Geometry check sheet. Reference: the model listing, model coordinates, mm. A direction names the side the tool comes from. Coordinates: 2 decimals unless noted, no trailing zeros. Write each loop counter-clockwise with the first axis right and the second up, starting at its lowest first coordinate (ties: lowest second). Pieces come first, ordered by that corner, then holes. Notation, with made-up numbers: (76, -8) -> (87, -8) arc R33 ccw to (87, 26) -> close; hole circle Ø8 at (52.5, 9.25). An arc over 180 degrees is marked (long way). Use a Markdown table: item, result.
```python
from build123d import *

# Parameters (mm, degrees)
SKETCH1_W               = 91.95
SKETCH1_H               = 32.25
BOSS_EXTRUDE1_DEPTH     = 3
SKETCH2_W               = 91.95
SKETCH2_H               = 2.15
CUT_EXTRUDE1_DEPTH      = 1.65
SKETCH4_W               = 3
SKETCH4_H               = 27.95
BOSS_EXTRUDE2_DEPTH     = 15
SKETCH5_R               = 1.25
CUT_EXTRUDE2_DEPTH      = 1
CUT_EXTRUDE2_DEPTH_BACK = 92.95
FILLET2_R               = 10
CUT_EXTRUDE5_REACH      = 20
SKETCH8_R               = 3
BOSS_EXTRUDE3_DEPTH     = 2
SKETCH9_R               = 1.25
CUT_EXTRUDE6_DEPTH      = 1
CUT_EXTRUDE6_DEPTH_BACK = 92.95


with BuildPart() as part:
    # Sketch1 → Boss-Extrude1 (new body)
    with BuildSketch(Plane(origin=(0, 0, 0), x_dir=(1, 0, 0), z_dir=(0, 1, 0))):
        with Locations((45.975, 16.125)):
            Rectangle(SKETCH1_W, SKETCH1_H)
    extrude(amount=BOSS_EXTRUDE1_DEPTH)

    # Sketch2 → Cut-Extrude1 (cut)
    with BuildSketch(Plane(origin=(0, 3, 0), x_dir=(1, 0, 0), z_dir=(0, 1, 0))):
        with Locations((45.975, 31.175)):
            Rectangle(SKETCH2_W, SKETCH2_H)
        with Locations((45.975, 1.075)):
            Rectangle(SKETCH2_W, SKETCH2_H)
    extrude(amount=-CUT_EXTRUDE1_DEPTH, mode=Mode.SUBTRACT)

    # Sketch4 → Boss-Extrude2 (add)
    with BuildSketch(Plane(origin=(0, 3, 0), x_dir=(1, 0, 0), z_dir=(0, 1, 0))):
        with Locations((1.5, 16.125)):
            Rectangle(SKETCH4_W, SKETCH4_H)
        with Locations((90.45, 16.125)):
            Rectangle(SKETCH4_W, SKETCH4_H)
    extrude(amount=BOSS_EXTRUDE2_DEPTH)

    # Sketch5 → Cut-Extrude2 (cut, two sides)
    with BuildSketch(Plane.ZY) as cut_extrude2_sk:
        with Locations((-17.25, 10)):
            Circle(SKETCH5_R)
    extrude(amount=CUT_EXTRUDE2_DEPTH, mode=Mode.SUBTRACT)
    extrude(cut_extrude2_sk.sketch, amount=-CUT_EXTRUDE2_DEPTH_BACK, mode=Mode.SUBTRACT)

    # Fillet2
    fillet2_edges = [part.edges().sort_by_distance(p)[0] for p in [
        (1.5, 18, -2.15),
        (1.5, 18, -30.1),
        (90.45, 18, -30.1),
        (90.45, 18, -2.15),
    ]]
    fillet(fillet2_edges, radius=FILLET2_R)

    # Sketch7 → Cut-Extrude5 (cut, up to next)
    with BuildSketch(Plane.XZ, mode=Mode.PRIVATE) as cut_extrude5_sk1:
        Polygon((7.95, -29.25), (10.95, -29.25), (6.321416756, -3), (3.321416756, -3), align=None)
    cut_extrude5_tool1 = extrude(cut_extrude5_sk1.sketch, amount=-CUT_EXTRUDE5_REACH, mode=Mode.PRIVATE) & part.part
    add(cut_extrude5_tool1.solids().sort_by_distance((7.135708, 0, -16.125))[0], mode=Mode.SUBTRACT)
    # Sketch7 → Cut-Extrude5 (cut, up to next)
    with BuildSketch(Plane.XZ, mode=Mode.PRIVATE) as cut_extrude5_sk2:
        Polygon((19.95, -29.25), (22.95, -29.25), (18.321416756, -3), (15.321416756, -3), align=None)
    cut_extrude5_tool2 = extrude(cut_extrude5_sk2.sketch, amount=-CUT_EXTRUDE5_REACH, mode=Mode.PRIVATE) & part.part
    add(cut_extrude5_tool2.solids().sort_by_distance((19.135708, 0, -16.125))[0], mode=Mode.SUBTRACT)
    # Sketch7 → Cut-Extrude5 (cut, up to next)
    with BuildSketch(Plane.XZ, mode=Mode.PRIVATE) as cut_extrude5_sk3:
        Polygon((25.95, -29.25), (28.95, -29.25), (24.321416756, -3), (21.321416756, -3), align=None)
    cut_extrude5_tool3 = extrude(cut_extrude5_sk3.sketch, amount=-CUT_EXTRUDE5_REACH, mode=Mode.PRIVATE) & part.part
    add(cut_extrude5_tool3.solids().sort_by_distance((25.135708, 0, -16.125))[0], mode=Mode.SUBTRACT)
    # Sketch7 → Cut-Extrude5 (cut, up to next)
    with BuildSketch(Plane.XZ, mode=Mode.PRIVATE) as cut_extrude5_sk4:
        Polygon((31.95, -29.25), (34.95, -29.25), (30.321416756, -3), (27.321416756, -3), align=None)
    cut_extrude5_tool4 = extrude(cut_extrude5_sk4.sketch, amount=-CUT_EXTRUDE5_REACH, mode=Mode.PRIVATE) & part.part
    add(cut_extrude5_tool4.solids().sort_by_distance((31.135708, 0, -16.125))[0], mode=Mode.SUBTRACT)
    # Sketch7 → Cut-Extrude5 (cut, up to next)
    with BuildSketch(Plane.XZ, mode=Mode.PRIVATE) as cut_extrude5_sk5:
        Polygon((37.95, -29.25), (40.95, -29.25), (36.321416756, -3), (33.321416756, -3), align=None)
    cut_extrude5_tool5 = extrude(cut_extrude5_sk5.sketch, amount=-CUT_EXTRUDE5_REACH, mode=Mode.PRIVATE) & part.part
    add(cut_extrude5_tool5.solids().sort_by_distance((37.135708, 0, -16.125))[0], mode=Mode.SUBTRACT)
    # Sketch7 → Cut-Extrude5 (cut, up to next)
    with BuildSketch(Plane.XZ, mode=Mode.PRIVATE) as cut_extrude5_sk6:
        Polygon((43.95, -29.25), (46.95, -29.25), (42.321416756, -3), (39.321416756, -3), align=None)
    cut_extrude5_tool6 = extrude(cut_extrude5_sk6.sketch, amount=-CUT_EXTRUDE5_REACH, mode=Mode.PRIVATE) & part.part
    add(cut_extrude5_tool6.solids().sort_by_distance((43.135708, 0, -16.125))[0], mode=Mode.SUBTRACT)
    # Sketch7 → Cut-Extrude5 (cut, up to next)
    with BuildSketch(Plane.XZ, mode=Mode.PRIVATE) as cut_extrude5_sk7:
        Polygon((55.95, -29.25), (58.95, -29.25), (54.321416756, -3), (51.321416756, -3), align=None)
    cut_extrude5_tool7 = extrude(cut_extrude5_sk7.sketch, amount=-CUT_EXTRUDE5_REACH, mode=Mode.PRIVATE) & part.part
    add(cut_extrude5_tool7.solids().sort_by_distance((55.135708, 0, -16.125))[0], mode=Mode.SUBTRACT)
    # Sketch7 → Cut-Extrude5 (cut, up to next)
    with BuildSketch(Plane.XZ, mode=Mode.PRIVATE) as cut_extrude5_sk8:
        Polygon((67.95, -29.25), (70.95, -29.25), (66.321416756, -3), (63.321416756, -3), align=None)
    cut_extrude5_tool8 = extrude(cut_extrude5_sk8.sketch, amount=-CUT_EXTRUDE5_REACH, mode=Mode.PRIVATE) & part.part
    add(cut_extrude5_tool8.solids().sort_by_distance((67.135708, 0, -16.125))[0], mode=Mode.SUBTRACT)
    # Sketch7 → Cut-Extrude5 (cut, up to next)
    with BuildSketch(Plane.XZ, mode=Mode.PRIVATE) as cut_extrude5_sk9:
        Polygon((79.95, -29.25), (75.321416756, -3), (78.321416756, -3), (82.95, -29.25), align=None)
    cut_extrude5_tool9 = extrude(cut_extrude5_sk9.sketch, amount=-CUT_EXTRUDE5_REACH, mode=Mode.PRIVATE) & part.part
    add(cut_extrude5_tool9.solids().sort_by_distance((79.135708, 0, -16.125))[0], mode=Mode.SUBTRACT)
    # Sketch7 → Cut-Extrude5 (cut, up to next)
    with BuildSketch(Plane.XZ, mode=Mode.PRIVATE) as cut_extrude5_sk10:
        Polygon((88.95, -29.25), (84.321416756, -3), (81.321416756, -3), (85.95, -29.25), align=None)
    cut_extrude5_tool10 = extrude(cut_extrude5_sk10.sketch, amount=-CUT_EXTRUDE5_REACH, mode=Mode.PRIVATE) & part.part
    add(cut_extrude5_tool10.solids().sort_by_distance((85.135708, 0, -16.125))[0], mode=Mode.SUBTRACT)
    # Sketch7 → Cut-Extrude5 (cut, up to next)
    with BuildSketch(Plane.XZ, mode=Mode.PRIVATE) as cut_extrude5_sk11:
        Polygon((16.95, -29.25), (12.321416756, -3), (9.321416756, -3), (13.95, -29.25), align=None)
    cut_extrude5_tool11 = extrude(cut_extrude5_sk11.sketch, amount=-CUT_EXTRUDE5_REACH, mode=Mode.PRIVATE) & part.part
    add(cut_extrude5_tool11.solids().sort_by_distance((13.135708, 0, -16.125))[0], mode=Mode.SUBTRACT)
    # Sketch7 → Cut-Extrude5 (cut, up to next)
    with BuildSketch(Plane.XZ, mode=Mode.PRIVATE) as cut_extrude5_sk12:
        Polygon((49.95, -29.25), (45.321416756, -3), (48.321416756, -3), (52.95, -29.25), align=None)
    cut_extrude5_tool12 = extrude(cut_extrude5_sk12.sketch, amount=-CUT_EXTRUDE5_REACH, mode=Mode.PRIVATE) & part.part
    add(cut_extrude5_tool12.solids().sort_by_distance((49.135708, 0, -16.125))[0], mode=Mode.SUBTRACT)
    # Sketch7 → Cut-Extrude5 (cut, up to next)
    with BuildSketch(Plane.XZ, mode=Mode.PRIVATE) as cut_extrude5_sk13:
        Polygon((61.95, -29.25), (57.321416756, -3), (60.321416756, -3), (64.95, -29.25), align=None)
    cut_extrude5_tool13 = extrude(cut_extrude5_sk13.sketch, amount=-CUT_EXTRUDE5_REACH, mode=Mode.PRIVATE) & part.part
    add(cut_extrude5_tool13.solids().sort_by_distance((61.135708, 0, -16.125))[0], mode=Mode.SUBTRACT)
    # Sketch7 → Cut-Extrude5 (cut, up to next)
    with BuildSketch(Plane.XZ, mode=Mode.PRIVATE) as cut_extrude5_sk14:
        Polygon((73.95, -29.25), (69.321416756, -3), (72.321416756, -3), (76.95, -29.25), align=None)
    cut_extrude5_tool14 = extrude(cut_extrude5_sk14.sketch, amount=-CUT_EXTRUDE5_REACH, mode=Mode.PRIVATE) & part.part
    add(cut_extrude5_tool14.solids().sort_by_distance((73.135708, 0, -16.125))[0], mode=Mode.SUBTRACT)

    # Sketch8 → Boss-Extrude3 (add)
    with BuildSketch(Plane(origin=(3, 0, 0), x_dir=(0, 0, -1), z_dir=(1, 0, 0))):
        with Locations((17.25, 10)):
            Circle(SKETCH8_R)
    boss_extrude3 = extrude(amount=BOSS_EXTRUDE3_DEPTH)

    # Mirror1: Boss-Extrude3 across plane
    add(boss_extrude3.mirror(Plane(origin=(45.975, 0, 0), x_dir=(0, 0, 1), z_dir=(1, 0, 0))))

    # Sketch9 → Cut-Extrude6 (cut, two sides)
    with BuildSketch(Plane.ZY) as cut_extrude6_sk:
        with Locations((-17.25, 10)):
            Circle(SKETCH9_R)
    extrude(amount=CUT_EXTRUDE6_DEPTH, mode=Mode.SUBTRACT)
    extrude(cut_extrude6_sk.sketch, amount=-CUT_EXTRUDE6_DEPTH_BACK, mode=Mode.SUBTRACT)


solid = part.part
```
Item 1: Tool access check on faces 4 (the flat face through (41.603, 1.479, -15.941)), 5 (the cylindrical face through (2.465, 11.054, -16.578)). Record the directions out of +Z, -Z, +X, -X, +Y, -Y that give a thin tool (end or side, any length) a straight path to the whole face; none if there is none.
Answer block:
| item | result |
|---|---|
| face 4 | +Y, -Y |
| face 5 | +X, -X |
Item 2: Mould release check, pull along Z, two halves, no side actions. Record for faces 1 (the flat face through (90, 18, -16)), 2 (the flat face through (17.603, 1.479, -15.941)), 3 (the cylindrical face through (87.964, 8.175, -14.869)): +Z half, -Z half, draft (parallel to the pull), parting line (faces both ways), or undercut.
Answer block:
| item | result |
|---|---|
| face 1 | draft |
| face 2 | undercut |
| face 3 | parting line |
Item 3: Section check B-B on y = 10. Record the boundary of the cut face in (x, z).
Answer block:
| item | result |
|---|---|
| outline | (0, -29.9) -> (3, -29.9) -> (3, -20.25) -> (5, -20.25) -> (5, -18.5) -> (0, -18.5) -> close; (0, -16) -> (5, -16) -> (5, -14.25) -> (3, -14.25) -> (3, -2.35) -> (0, -2.35) -> close; (86.95, -20.25) -> (88.95, -20.25) -> (88.95, -29.9) -> (91.95, -29.9) -> (91.95, -18.5) -> (86.95, -18.5) -> close; (86.95, -16) -> (91.95, -16) -> (91.95, -2.35) -> (88.95, -2.35) -> (88.95, -14.25) -> (86.95, -14.25) -> close |
Item 4: Section check A-A on y = 15. Record the boundary of the cut face in (x, z).
Answer block:
| item | result |
|---|---|
| outline | (0, -27.24) -> (3, -27.24) -> (3, -5.01) -> (0, -5.01) -> close; (88.95, -27.24) -> (91.95, -27.24) -> (91.95, -5.01) -> (88.95, -5.01) -> close |
Item 5: Thickness scan on L1, parallel to Y at x = 1.4, z = -17.25; L2, parallel to X at y = 7.25, z = -3; L3, parallel to Y at x = 23.5, z = -23. Record the ranges inside material, lowest first. Write a range as [from, to].
Answer block:
| item | result |
|---|---|
| L1 | y = [0, 8.75], [11.25, 18] |
| L2 | x = [0, 3], [88.95, 91.95] |
| L3 | y = [0, 3] |
Item 6: Depth check by flat-ended pin: P1, Ø3, axis at x = 50, z = -19, coming from the -Y side; P2, Ø0.9, axis at x = 71, y = 2, coming from the -Z side; P3, Ø6, axis at x = 36, z = -16.5, coming from the +Y side; P4, Ø2, axis at y = 10, z = -17.25, coming from the -X side. Enter the tip coordinate at first touch or a pass-through.
Answer block:
| item | result |
|---|---|
| P1 | stops at y = 0 |
| P2 | stops at z = -30.1 |
| P3 | stops at y = 3 |
| P4 | passes through |
Item 7: Section check C-C on z = -17.25. Count the separate pieces of the cut face and the enclosed holes in it, then the cut area to 3 significant figures.
Answer block:
| item | result |
|---|---|
| separate pieces | 17 |
| enclosed holes | 0 |
| area | 239 mm^2 |
